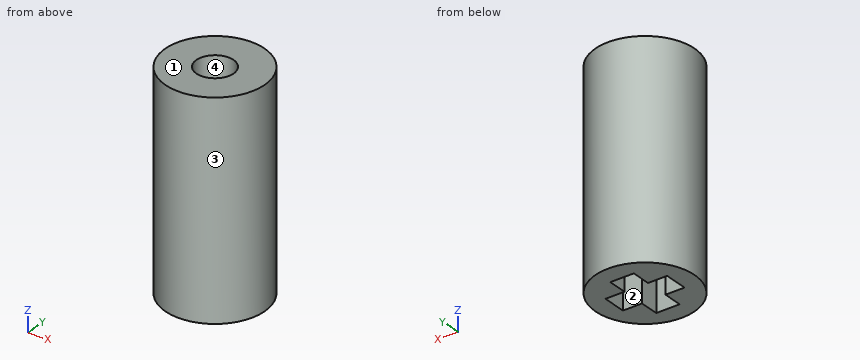
```python
from build123d import *

# Parameters (mm, degrees)
SKETCH004_R     = 4
PAD002_DEPTH    = 17
SKETCH005_R     = 1.5
POCKET002_DEPTH = 8
POCKET003_DEPTH = 8


with BuildPart() as part:
    # Sketch004 → Pad002 (new body)
    with BuildSketch(Plane.XY):
        Circle(SKETCH004_R)
    extrude(amount=PAD002_DEPTH)

    # Sketch005 → Pocket002 (cut)
    with BuildSketch(Plane.XY.offset(17)):
        Circle(SKETCH005_R)
    extrude(amount=-POCKET002_DEPTH, mode=Mode.SUBTRACT)

    # Sketch006 → Pocket003 (cut)
    with BuildSketch(Plane(origin=(0, 0, 0), x_dir=(1, 0, 0), z_dir=(0, 0, -1))):
        Polygon((-0.95, 2.5), (0.95, 2.5), (0.95, 0.95), (2.5, 0.95), (2.5, -0.95), (0.95, -0.95), (0.95, -2.5), (-0.95, -2.5), (-0.95, -0.95), (-2.5, -0.95), (-2.5, 0.95), (-0.95, 0.95), align=None)
    extrude(amount=-POCKET003_DEPTH, mode=Mode.SUBTRACT)


solid = part.part
```
Read the model definition and answer for the solid it produces. Units are mm, in the model's axes. Face numbers are marked on the shaded views. Round coordinates to 2 decimals unless told otherwise and drop trailing zeros. Write each loop counter-clockwise with the first axis right and the second up, starting at its lowest first coordinate (ties: lowest second). Pieces come first, ordered by that corner, then holes. Notation, with made-up numbers: M -11,-13.75 L 30,-13.75 A20 ccw 30,-6.75 Z; hole C 2,-38 d1. An arc over 180 degrees is marked long. One line per item, written item: value.
Q1. For a pull along X with two mould halves and no side action, classify the marked faces 1, 2, 3 and 4 as +X half, -X half, draft (parallel to the pull), parting line (faces both ways), or undercut.
Data:
face 1: draft
face 2: undercut
face 3: parting line
face 4: undercut
Q2. Straight lines are drawn through the part: line 1 (Y direction, x = 0, z = 13.25); line 2 (Y direction, x = -0.5, z = 15); line 3 (Z direction, x = 1.25, y = 0). For each, find the intervals that lie inside material, in ascending order. Write a range as [from, to].
Data:
line 1: [-4, -1.5], [1.5, 4]
line 2: [-3.97, -1.41], [1.41, 3.97]
line 3: [8, 9]
Q3. Find section A-A on z = 7.5. Write down the section's boundary in (x, y).
Data:
outline: C 0,0 d8; hole M -2.5,-0.95 L -0.95,-0.95 L -0.95,-2.5 L 0.95,-2.5 L 0.95,-0.95 L 2.5,-0.95 L 2.5,0.95 L 0.95,0.95 L 0.95,2.5 L -0.95,2.5 L -0.95,0.95 L -2.5,0.95 Z
Q4. Find section D-D on x = 1.75. Write down the section's boundary in (y, z), plus the area to 3 significant figures.
Data:
outline: M -3.6,0 L -0.95,0 L -0.95,8 L 0.95,8 L 0.95,0 L 3.6,0 L 3.6,17 L -3.6,17 Z
area: 107 mm2
Q5. Flat-ended cylindrical pins translate along their axes: pin 1 Ø1.2 at (x, z) = (2, 5) entering from +Y; pin 2 Ø0.5 at (y, z) = (1.5, 4.5) entering from -X; pin 3 Ø2.5 at (x, y) = (0.5, 0.5) entering from -Z; pin 4 Ø1.7 at (x, z) = (-2, 2) entering from -Y. Find the tip coordinate at first contact, or state that the pin passes through.
Data:
pin 1: y = 3.75
pin 2: x = -3.8
pin 3: z = 0
pin 4: y = -3.83
Q6. Find section B-B on y = 0. Write down the section's boundary in (x, z), plus the area to 3 significant figures.
Data:
outline: M -4,0 L -2.5,0 L -2.5,8 L 2.5,8 L 2.5,0 L 4,0 L 4,17 L 1.5,17 L 1.5,9 L -1.5,9 L -1.5,17 L -4,17 Z
area: 72.0 mm2
